```python
from build123d import *

# Parameters (mm, degrees)
F0_W     = 15
F0_H     = 80
F3_DEPTH = 5


with BuildPart() as f1:
    # F0 (on Front) → F1 (revolve)
    with BuildSketch(Plane.XZ):
        with Locations((-7.5, 40)):
            Rectangle(F0_W, F0_H)
    revolve(axis=Axis((0, 0, 40), (0, 0, 1)))

    # F2 (on face) → F3 (cut)
    with BuildSketch(Plane.XY.offset(80)):
        with BuildLine():
            ThreePointArc((3, 14.6969384567), (0, 15), (-3, 14.6969384567))
            Line((-3, 14.6969384567), (-3, -14.6969384567))
            ThreePointArc((-3, -14.6969384567), (0, -15), (3, -14.6969384567))
            Line((3, -14.6969384567), (3, 14.6969384567))
        make_face()
    extrude(amount=-F3_DEPTH, mode=Mode.SUBTRACT)


solid = f1.part
```
Geometry check sheet. Reference: the model listing, model coordinates, mm. A direction names the side the tool comes from. Give positions to 0.01 mm unless a question says otherwise; leave off trailing zeros. Write each loop counter-clockwise with the first axis right and the second up, starting at its lowest first coordinate (ties: lowest second). Pieces come first, ordered by that corner, then holes. Notation, with made-up numbers: (-24.5, 39.25) - (13.5, 39.25) arc R25 ccw to (13.5, 57.25) - close; hole circle Ø5 at (52.5, 48.5). An arc over 180 degrees is marked (long way). Use a Markdown table: item, result.
Q1. Draft check along X on faces 3 (the face through (-3, 0, 78)), 4 (the face through (8, 0, 80)), 5 (the face through (3, 0, 78)), 6 (the face through (3.252, 14.643, 40.56)). Enter one of: pulls with the +X half, pulls with the -X half, needs draft (parallel to the pull), parting line crosses it, or undercut.
Computed:
| item | result |
|---|---|
| face 3 | undercut |
| face 4 | needs draft |
| face 5 | undercut |
| face 6 | parting line crosses it |
Q2. Section check D-D, the plane y = -6.5. Enter the section's corners in (x, z).
Computed:
| item | result |
|---|---|
| outline | (-13.52, 0) - (13.52, 0) - (13.52, 80) - (3, 80) - (3, 75) - (-3, 75) - (-3, 80) - (-13.52, 80) - close |
Q3. Section check B-B, the plane z = 57.5. Enter the section's corners in (x, y), then the cut area to 3 significant figures.
Computed:
| item | result |
|---|---|
| outline | circle Ø30 at (0, 0) |
| area | 707 mm² |
Q4. Go/stop test with flat-tipped pins: P1, Ø8, axis at x = -11, z = 39.5, coming from the +Y side; P2, Ø2, axis at x = 9, z = 68, coming from the -Y side; P3, Ø2.5, axis at y = 7.5, z = 77.5, coming from the -X side. Record where each tip stops, or that it passes through.
Computed:
| item | result |
|---|---|
| P1 | stops at y = 13.27 |
| P2 | stops at y = -12.69 |
| P3 | stops at x = -13.64 |
Q5. Section check A-A, the plane y = 1.25. Enter the section's corners in (x, z), then the cut area to 3 significant figures.
Computed:
| item | result |
|---|---|
| outline | (-14.95, 0) - (14.95, 0) - (14.95, 80) - (3, 80) - (3, 75) - (-3, 75) - (-3, 80) - (-14.95, 80) - close |
| area | 2,360 mm² |
Q6. Set-up check for faces 1 (the face through (0, 0, 0)), 2 (the face through (0, 0, 75)): record each of +Z, -Z, +X, -X, +Y, -Y from which the full face is reachable in a straight line by a thin tool's end or side.
Computed:
| item | result |
|---|---|
| face 1 | -Z, +X, -X, +Y, -Y |
| face 2 | +Z, +Y, -Y |
Q7. Thickness scan on L1, parallel to Y at x = -0.5, z = 67.5; L2, parallel to Y at x = -7.5, z = 36; L3, parallel to X at y = 5.25, z = 18. Record the ranges inside material, lowest first. Write a range as [from, to].
Computed:
| item | result |
|---|---|
| L1 | y = [-14.99, 14.99] |
| L2 | y = [-12.99, 12.99] |
| L3 | x = [-14.05, 14.05] |
Q8. Section check C-C, the plane x = 12. Enter the section's corners in (y, z), then the cut area to 3 significant figures.
Computed:
| item | result |
|---|---|
| outline | (-9, 0) - (9, 0) - (9, 80) - (-9, 80) - close |
| area | 1,440 mm² |
